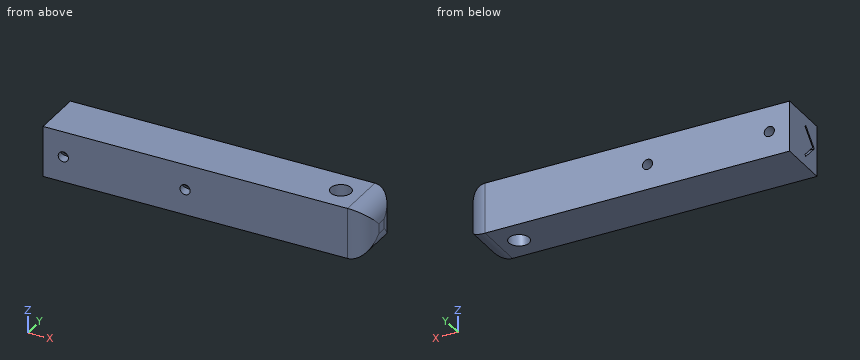
```python
from build123d import *

# Parameters (mm, degrees)
BOSS_EXTRUDE1_DEPTH         = 15.875
CUT_EXTRUDE1_DEPTH          = 152.4
F_1_2_0_5_DIAMETER_HOLE1_D  = 12.7
F_1_4_0_25_DIAMETER_HOLE1_D = 6.35
FILLET1_R                   = 12.7


with BuildPart() as part:
    # Sketch1 → Boss-Extrude1 (new, symmetric)
    with BuildSketch(Plane.XY):
        Polygon((0, 0), (101.6, 0), (101.6, 31.75), (-101.6, 31.75), (-101.6, 0), align=None)
    extrude(amount=BOSS_EXTRUDE1_DEPTH, both=True)

    # Sketch2 → Cut-Extrude1 (cut)
    with BuildSketch(Plane.ZY.offset(101.6)):
        Polygon((0, 4.971051224), (-8.980256121, 13.951307345), (-9.878281733, 13.053281733), (0, 3.175), (9.878281733, 13.053281733), (8.980256121, 13.951307345), align=None)
    extrude(amount=-CUT_EXTRUDE1_DEPTH, mode=Mode.SUBTRACT)

    # 1/2 (0.5) Diameter Hole1 (through all)
    with Locations(Plane.XY.offset(15.875)):
        with Locations((76.2, 15.875)):
            Hole(F_1_2_0_5_DIAMETER_HOLE1_D / 2)

    # 1/4 (0.25) Diameter Hole1 (through all)
    with Locations(Plane(origin=(0, 31.75, 0), x_dir=(1, 0, 0), z_dir=(0, 1, 0))):
        with Locations((-88.9, 0), (-12.7, 0)):
            Hole(F_1_4_0_25_DIAMETER_HOLE1_D / 2)

    # Fillet1
    fillet1_edges = [part.edges().sort_by_distance(p)[0] for p in [
        (101.6, 15.875, 15.875),
        (101.6, 15.875, -15.875),
        (101.6, 31.75, 0),
        (101.6, 0, 0),
    ]]
    fillet(fillet1_edges, radius=FILLET1_R)


solid = part.part
```
Could you check a few things on this model? Use its own coordinates, in mm. Round coordinates to 2 decimals unless told otherwise and drop trailing zeros. Loops run counter-clockwise (first coordinate to the right, second up) from the corner with the lowest first, then second, coordinate; pieces in that order, holes last.
Q1. I want a section at C-C (y = 27.5). Write out the boundary of the cut face in (x, z) (3 decimals).
Q2. Please list where these lines run through material, in increasing order: L1, parallel to Z at x = -20, y = 13 (3 decimals); L2, parallel to Z at x = 21, y = 10 (3 decimals); L3, parallel to Y at x = 76.2, z = -7 (3 decimals).
Q3. I want a section at A-A (x = 76.2). Write out the boundary of the cut face in (y, z) (3 decimals).
Q4. I want a section at D-D (x = -12.7). Write out the boundary of the cut face in (y, z) (3 decimals).
Q5. I want a section at B-B (z = 6). Write out the boundary of the cut face in (x, y) (3 decimals).
Q6. For P1, Ø5.5, axis at x = -88.9, z = 0, coming from the -Y side; P2, Ø8.5, axis at x = -12.7, z = 0, coming from the -Y side, each with a flat end and sliding along its axis, tell me the tip position at first contact or that it passes through.
Answer below:
1. outline: (-101.6, -15.875) - (88.9, -15.875) arc R12.7 ccw to (98.381, -11.625) - (98.381, 11.625) arc R12.7 ccw to (88.9, 15.875) - (-101.6, 15.875) - close; hole circle Ø6.35 at (-88.9, 0); hole circle Ø6.35 at (-12.7, 0)
2. L1: z = -15.875 to -9.825, -8.029 to 8.029, 9.825 to 15.875
2. L2: z = -15.875 to -6.825, -5.029 to 5.029, 6.825 to 15.875
2. L3: y = 0 to 9.525, 22.225 to 31.75
3. outline: (0, -15.875) - (9.525, -15.875) - (9.525, 15.875) - (0, 15.875) - close; (22.225, -15.875) - (31.75, -15.875) - (31.75, 15.875) - (22.225, 15.875) - close
4. outline: (0, -15.875) - (31.75, -15.875) - (31.75, -3.175) - (8.146, -3.175) - (13.951, -8.98) - (13.053, -9.878) - (6.35, -3.175) - (0, -3.175) - close; (0, 3.175) - (6.35, 3.175) - (13.053, 9.878) - (13.951, 8.98) - (8.146, 3.175) - (31.75, 3.175) - (31.75, 15.875) - (0, 15.875) - close
5. outline: (-101.6, 0) - (88.9, 0) arc R12.7 ccw to (101.282, 9.875) - (101.282, 21.875) arc R12.7 ccw to (88.9, 31.75) - (-101.6, 31.75) - (-101.6, 10.971) - (50.8, 10.971) - (50.8, 9.175) - (-101.6, 9.175) - close; hole circle Ø12.7 at (76.2, 15.875)
6. P1: passes through
6. P2: stops at y = 0
